For this review, take the finished solid that the model builds, in its own axes (mm). Coordinates: 2 decimals unless noted, no trailing zeros. Write each loop counter-clockwise with the first axis right and the second up, starting at its lowest first coordinate (ties: lowest second). Pieces come first, ordered by that corner, then holes.
1) We need section B-B on x = 259.5. Write out the cut boundary in (y, z).
2) To check wall thickness, follow line 1 along X through (y, z) = (162, 12.75); line 2 along Y through (x, z) = (44, 6); line 3 along Y through (x, z) = (604.5, 8.75). State the ranges of each line that lie inside material, in increasing order.
3) We need section C-C on y = 263. Write out the cut boundary in (x, z), then the cut area to 3 significant figures.
4) Insertion check: P1, Ø6, axis at x = -489, z = 15.5, coming from the -Y side; P2, Ø5.5, axis at y = 270, z = 7, coming from the +X side; P3, Ø1, axis at y = 181, z = 12, coming from the -X side. Each pin has a flat end and moves straight along its axis. Give the tip position at first contact, or say it passes through.
5) We need section A-A on z = 14. Write out the cut boundary in (x, y).
from build123d import *

# Parameters (mm, degrees)
F1_DEPTH = 18
F3_DEPTH = 2000


with BuildPart() as f1:
    # F0 (on Top) → F1 (new body)
    with BuildSketch(Plane.XY):
        Polygon((1000, -150), (1000, 150), (700, 150), (700, 450), (-700, 450), (-700, 150), (-1000, 150), (-1000, -150), align=None)
    extrude(amount=F1_DEPTH)

    # F2 (on face) → F3 (cut)
    with BuildSketch(Plane.YZ.offset(1000)):
        Polygon((-132, 0), (-150, 18), (-150, 0), align=None)
    extrude(amount=-F3_DEPTH, mode=Mode.SUBTRACT)


solid = f1.part
Result:
1. outline: (-150, 18) - (-132, 0) - (450, 0) - (450, 18) - close
2. line 1: x = -700 to 700
2. line 2: y = -138 to 450
2. line 3: y = -140.75 to 450
3. outline: (-700, 0) - (700, 0) - (700, 18) - (-700, 18) - close
3. area: 25,200 mm2
4. P1: stops at y = -150
4. P2: stops at x = 700
4. P3: stops at x = -700
5. outline: (-1000, -146) - (1000, -146) - (1000, 150) - (700, 150) - (700, 450) - (-700, 450) - (-700, 150) - (-1000, 150) - close
